Source: three-view drawing plus pictorial views. Frame: mm from the lowest corner of the part. Give positions to 0.01 mm unless a question says otherwise; leave off trailing zeros. Loops run counter-clockwise (first coordinate to the right, second up) from the corner with the lowest first, then second, coordinate; pieces in that order, holes last.
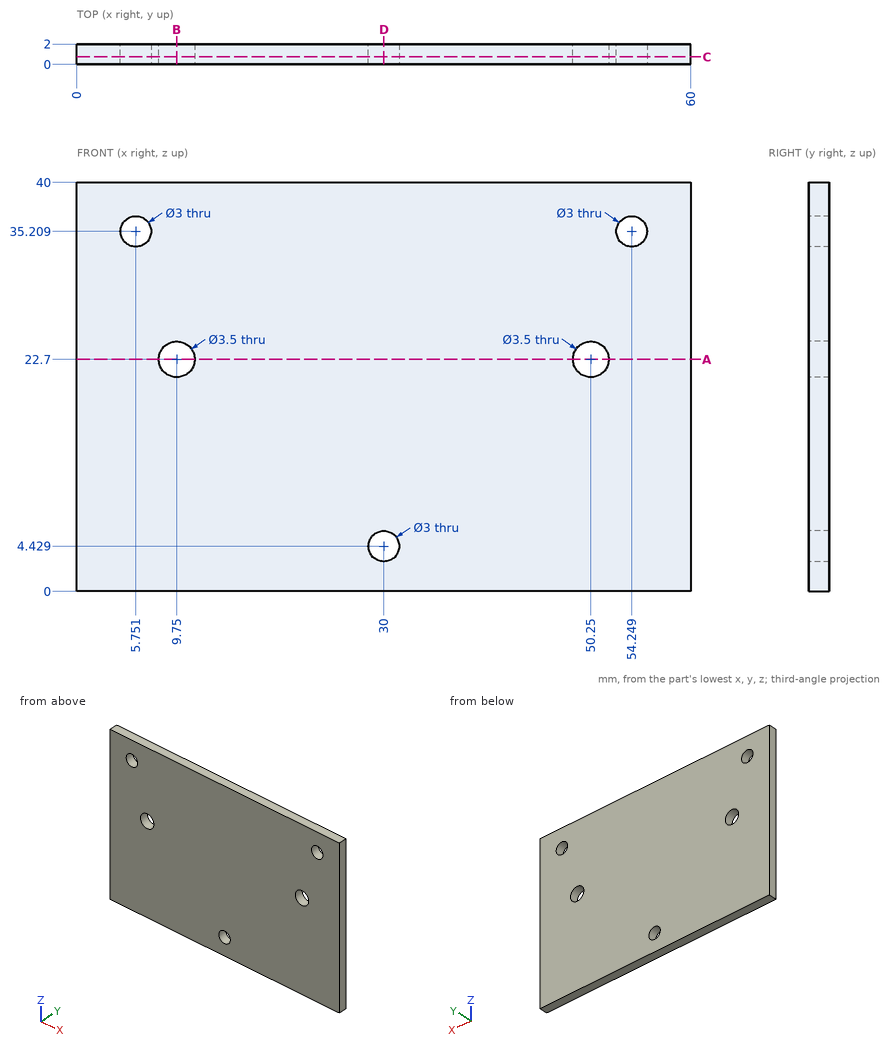
1) Cut plane C-C (y = 0.75). Return loops of the section in (x, z).
Checks:
outline: (0, 0) - (60, 0) - (60, 40) - (0, 40) - close; hole circle Ø3 at (5.75, 35.21); hole circle Ø3.5 at (9.75, 22.7); hole circle Ø3 at (30, 4.43); hole circle Ø3.5 at (50.25, 22.7); hole circle Ø3 at (54.25, 35.21)
2) Cut plane A-A (z = 22.7). Return loops of the section in (x, y).
Checks:
outline: (0, 0) - (8, 0) - (8, 2) - (0, 2) - close; (11.5, 0) - (48.5, 0) - (48.5, 2) - (11.5, 2) - close; (52, 0) - (60, 0) - (60, 2) - (52, 2) - close
3) Ray query, probe 1 along Z at (x, y) = (50.25, 1.4); probe 2 along Z at (x, y) = (30, 1.05); probe 3 along X at (y, z) = (0.7, 23) (1 decimal). Return the intervals inside material, ascending.
Checks:
probe 1: z = 0 to 20.95, 24.45 to 40
probe 2: z = 0 to 2.93, 5.93 to 40
probe 3: x = 0 to 8, 11.5 to 48.5, 52 to 60
4) Cut plane B-B (x = 9.75). Return loops of the section in (y, z).
Checks:
outline: (0, 0) - (2, 0) - (2, 20.95) - (0, 20.95) - close; (0, 24.45) - (2, 24.45) - (2, 40) - (0, 40) - close
5) Cut plane D-D (x = 30). Return loops of the section in (y, z).
Checks:
outline: (0, 0) - (2, 0) - (2, 2.93) - (0, 2.93) - close; (0, 5.93) - (2, 5.93) - (2, 40) - (0, 40) - close
